```python
from build123d import *

# Parameters (mm, degrees)
SKETCH1_W           = 210
SKETCH1_H           = 50
SKETCH1_R           = 1.211665018
SKETCH1_R_2         = 1.165617118
SKETCH1_R_3         = 1.5
SKETCH1_R_4         = 1.25
SKETCH1_R_5         = 1.517273905
BOSS_EXTRUDE1_DEPTH = 3.175
SKETCH2_R           = 2
CUT_EXTRUDE1_DEPTH  = 10
SKETCH3_R           = 6
SKETCH3_R_2         = 0.586995366
CUT_EXTRUDE2_DEPTH  = 57.15
CUT_EXTRUDE7_DEPTH  = 10
FILLET3_R           = 5
SKETCH11_R          = 18.5
SKETCH11_R_2        = 2
BOSS_EXTRUDE4_DEPTH = 3.175
SKETCH16_W          = 18.257640281
SKETCH16_H          = 3.175
BOSS_EXTRUDE7_DEPTH = 8.128
SKETCH17_W          = 33.3
SKETCH17_H          = 3.175
BOSS_EXTRUDE8_DEPTH = 35.56
SKETCH18_R          = 2
CUT_EXTRUDE8_DEPTH  = 9
SKETCH19_R          = 4
CUT_EXTRUDE9_DEPTH  = 40
FILLET4_R           = 5


with BuildPart() as part:
    # Sketch1 → Boss-Extrude1 (new body)
    with BuildSketch(Plane(origin=(0, 0, 0), x_dir=(1, 0, 0), z_dir=(0, 1, 0))):
        with Locations((105, -25)):
            Rectangle(SKETCH1_W, SKETCH1_H)
        with Locations(Location((3.489526233, -16.787661112, 0), (0, 0, 270))):
            Circle(SKETCH1_R, mode=Mode.SUBTRACT)
        with Locations(Location((34.37258772, -17.194005245, 0), (0, 0, 270))):
            Circle(SKETCH1_R_2, mode=Mode.SUBTRACT)
        with Locations(Location((37.520749958, -44.921198121, 0), (0, 0, 270))):
            Circle(SKETCH1_R_3, mode=Mode.SUBTRACT)
        with Locations(Location((118.879039361, -40.017685043, 0), (0, 0, 270))):
            Circle(SKETCH1_R_4, mode=Mode.SUBTRACT)
        with Locations(Location((112.302052499, -4.739260115, 0), (0, 0, 270))):
            Circle(SKETCH1_R_3, mode=Mode.SUBTRACT)
        with Locations(Location((168.975233936, -37.403209633, 0), (0, 0, 270))):
            Circle(SKETCH1_R_5, mode=Mode.SUBTRACT)
    extrude(amount=BOSS_EXTRUDE1_DEPTH)

    # Sketch2 → Cut-Extrude1 (cut)
    with BuildSketch(Plane(origin=(0, 3.175, 0), x_dir=(1, 0, 0), z_dir=(0, 1, 0))):
        with Locations(Location((10, -26, 0), (0, 0, 270))):
            Circle(SKETCH2_R)
        with Locations(Location((10, -42, 0), (0, 0, 270))):
            Circle(SKETCH2_R)
        with Locations(Location((26, -26, 0), (0, 0, 270))):
            Circle(SKETCH2_R)
        with Locations(Location((26, -42, 0), (0, 0, 270))):
            Circle(SKETCH2_R)
    extrude(amount=-CUT_EXTRUDE1_DEPTH, mode=Mode.SUBTRACT)

    # Sketch3 → Cut-Extrude2 (cut)
    with BuildSketch(Plane(origin=(0, 3.175, 0), x_dir=(1, 0, 0), z_dir=(0, 1, 0))):
        with Locations(Location((78.01026379, -28.1, 0), (0, 0, 270))):
            Circle(SKETCH3_R)
        with Locations(Location((145.531297368, -14, 0), (0, 0, 270))):
            Circle(SKETCH3_R)
        with Locations(Location((18, -34, 0), (0, 0, 270))):
            Circle(SKETCH3_R_2)
        with Locations(Location((202.646291021, -16, 0), (0, 0, 270))):
            Circle(SKETCH3_R)
    extrude(amount=-CUT_EXTRUDE2_DEPTH, mode=Mode.SUBTRACT)

    # Sketch10 → Cut-Extrude7 (cut)
    with BuildSketch(Plane(origin=(0, 3.175, 0), x_dir=(1, 0, 0), z_dir=(0, 1, 0))):
        Polygon((210, -27.859435908), (165.502877994, -50), (210, -50), align=None)
        Polygon((92.532613397, 0), (77.65477062, -7.402812063), (0, -7.402812063), (0, 0), align=None)
    extrude(amount=-CUT_EXTRUDE7_DEPTH, mode=Mode.SUBTRACT)

    # Fillet3
    fillet3_edges = [part.edges().sort_by_distance(p)[0] for p in [
        (210, 1.5875, 0),
        (92.532613397, 1.5875, 0),
        (210, 1.5875, 27.859435908),
        (165.502877994, 1.5875, 50),
        (77.65477062, 1.5875, 7.402812063),
    ]]
    fillet(fillet3_edges, radius=FILLET3_R)

    # Sketch11 → Boss-Extrude4 (add)
    with BuildSketch(Plane(origin=(0, 3.175, 0), x_dir=(1, 0, 0), z_dir=(0, 1, 0))):
        with Locations((18, -34)):
            Circle(SKETCH11_R)
        with Locations(Location((10, -26, 0), (0, 0, 270))):
            Circle(SKETCH11_R_2, mode=Mode.SUBTRACT)
        with Locations(Location((10, -42, 0), (0, 0, 270))):
            Circle(SKETCH11_R_2, mode=Mode.SUBTRACT)
        with Locations(Location((26, -26, 0), (0, 0, 270))):
            Circle(SKETCH11_R_2, mode=Mode.SUBTRACT)
        with Locations(Location((26, -42, 0), (0, 0, 270))):
            Circle(SKETCH11_R_2, mode=Mode.SUBTRACT)
    extrude(amount=-BOSS_EXTRUDE4_DEPTH)

    # Sketch16 → Boss-Extrude7 (add)
    with BuildSketch(Plane(origin=(0, 0, 7.402812063), x_dir=(-1, 0, 0), z_dir=(0, 0, -1))):
        with Locations((-9.128820141, 1.5875)):
            Rectangle(SKETCH16_W, SKETCH16_H)
    extrude(amount=BOSS_EXTRUDE7_DEPTH)

    # Sketch17 → Boss-Extrude8 (add)
    with BuildSketch(Plane.ZY):
        with Locations((15.924812063, 1.5875)):
            Rectangle(SKETCH17_W, SKETCH17_H)
    extrude(amount=BOSS_EXTRUDE8_DEPTH)

    # Sketch18 → Cut-Extrude8 (cut)
    with BuildSketch(Plane(origin=(0, 3.175, 0), x_dir=(1, 0, 0), z_dir=(0, 1, 0))):
        with Locations(Location((-29.612034681, -23.798543698, 0), (0, 0, 270))):
            Circle(SKETCH18_R)
        with Locations(Location((-29.359661767, -7.798707515, 0), (0, 0, 270))):
            Circle(SKETCH18_R)
        with Locations(Location((-13.359825583, -8.051080428, 0), (0, 0, 270))):
            Circle(SKETCH18_R)
        with Locations(Location((-13.612198497, -24.050916612, 0), (0, 0, 270))):
            Circle(SKETCH18_R)
    extrude(amount=-CUT_EXTRUDE8_DEPTH, mode=Mode.SUBTRACT)

    # Sketch19 → Cut-Extrude9 (cut)
    with BuildSketch(Plane(origin=(0, 3.175, 0), x_dir=(1, 0, 0), z_dir=(0, 1, 0))):
        with Locations(Location((-21.359661767, -15.798707515, 0), (0, 0, 270))):
            Circle(SKETCH19_R)
    extrude(amount=-CUT_EXTRUDE9_DEPTH, mode=Mode.SUBTRACT)

    # Fillet4
    fillet4_edges = [part.edges().sort_by_distance(p)[0] for p in [
        (18.257640281, 1.5875, -0.725187937),
        (-35.56, 1.5875, -0.725187937),
        (-35.56, 1.5875, 32.574812063),
        (0, 1.5875, 50),
    ]]
    fillet(fillet4_edges, radius=FILLET4_R)


solid = part.part
```
Could you check a few things on this model? Use its own coordinates, in mm. A direction names the side the tool comes from. Round coordinates to 2 decimals unless told otherwise and drop trailing zeros. Write each loop counter-clockwise with the first axis right and the second up, starting at its lowest first coordinate (ties: lowest second). Pieces come first, ordered by that corner, then holes. Notation, with made-up numbers: M -14,58.25 L 45,58.25 A10 ccw 45,76.25 Z; hole C -34.75,89 d8. An arc over 180 degrees is marked long. Answer in a Markdown table with one row per item. Add a question column.
Q1. On a 3-axis mill with a long thin cutter (end or side, diameter ignored), from which of +Z, -Z, +X, -X, +Y, -Y can I reach the whole of each face in a straight line? I mean faces 1 (the flat face through (187.176, 1.61, 39.216)), 2 (the flat face through (85.18, 1.61, 3.66)). Say none if no direction works.
Q2. Imagine slicing it at A-A (x = 124). Please give me the cut outline in (y, z) (3 decimals).
Q3. If I drill on line 1 (X direction, y = 1.4, z = 41); line 2 (Z direction, x = 145, y = 0.3); line 3 (X direction, y = 1.7, z = 14), over which ranges is the centre line in solid material (lowest first)? Write a range as from..to.
Q4. Imagine slicing it at B-B (y = 2.6). Give the number of separate pieces and of enclosed holes in the cut face, then the cut area to 3 significant figures.
Q5. If we mould it in two halves opening along X, with no side actions, what happens to faces 3 (the cylindrical face through (16.754, 1.61, 0.701)), 4 (the cylindrical face through (-34.134, 1.61, 31.071)), 5 (the cylindrical face through (208, 2, 1)), 6 (the flat face through (89, 3.175, 26))? For each: +X half, -X half, draft (parallel to the pull), parting line (faces both ways), or undercut.
Q6. Will these pins go through, and if not, where does the flat tip stop? pin 1 Ø1 at (x, y) = (44, 1.5) entering from -Z; pin 2 Ø1.5 at (y, z) = (2, 45) entering from +X; pin 3 Ø1.6 at (x, y) = (81, 1.5) entering from +Z.
Q7. Imagine slicing it at C-C (x = 175.5). Please give me the cut outline in (y, z) (3 decimals).
Values:
| question | item | result |
|---|---|---|
| 1 | face 1 | +Z, +X, +Y, -Y |
| 1 | face 2 | -Z, +Y, -Y |
| 2 | outline | M 0,0 L 3.175,0 L 3.175,50 L 0,50 Z |
| 3 | line 1 | 0..8.27, 11.73..24.27, 27.73..118.11, 119.65..183.59 |
| 3 | line 2 | 0..8.02, 19.98..50 |
| 3 | line 3 | -35.56..-24.93, -17.79..139.53, 151.53..196.99, 208.3..210 |
| 4 | separate pieces | 1 |
| 4 | enclosed holes | 18 |
| 4 | area | 10,200 mm^2 |
| 5 | face 3 | undercut |
| 5 | face 4 | -X half |
| 5 | face 5 | +X half |
| 5 | face 6 | draft |
| 6 | pin 1 | z = 7.4 |
| 6 | pin 2 | x = 177.06 |
| 6 | pin 3 | z = 50 |
| 7 | outline | M 0,0 L 3.175,0 L 3.175,45.026 L 0,45.026 Z |
